Geometry: final body of the model. Coordinates: model frame, mm. Round coordinates to 2 decimals unless told otherwise and drop trailing zeros. Order: outer loops, then holes, each group sorted by start corner. A loop starts at its lowest first (then second) coordinate and runs counter-clockwise, first axis right, second up. Notation, with made-up numbers: M 1.5,11 L 43.5,11 A27 cw 43.5,34 Z; hole C 49.5,25 d1. An arc over 180 degrees is marked long. Return JSON: item names as keys, results as strings. Group by question number.
Q1. Cut plane A-A on z = 285. Output: boundary loops of the cut face in (x, y), and give its area (3 significant figures).
Q2. Ray query, probe 1 along Y at (x, z) = (0, 188.5); probe 2 along Y at (x, z) = (-0.5, 73). Return the intervals inside material, ascending.
Q3. Contact query for flat-ended pins moving along their axis: pin 1 (1.7 mm diameter, centred on x = -3.5, y = 2, fed in from +Z); pin 2 (1.5 mm diameter, centred on x = 0, y = 3.5, fed in from +Z); pin 3 (2.5 mm diameter, centred on y = 0, z = 5.5, fed in from +X); pin 4 (4 mm diameter, centred on y = -2, z = 220.5, fed in from +X). Output: stop coordinate, or through.
```python
from build123d import *
from build123d.topology import SkipClean

# Parameters (mm, degrees)
SKETCH_1_R          = 2.5
EXTRUDE_1_DEPTH     = 345
CUT_EXTRUDE_1_DEPTH = 4.8
SKETCH_3_R          = 5
SKETCH_3_R_2        = 2.75
EXTRUDE_2_DEPTH     = 290
SKETCH_4_R          = 5
EXTRUDE_3_DEPTH     = 5
CUT_EXTRUDE_START   = -5
CUT_EXTRUDE_2_DEPTH = 5


with BuildPart() as part:
    # Sketch 1 → Extrude 1 (new body)
    with BuildSketch(Plane.XY):
        Circle(SKETCH_1_R)
    extrude(amount=EXTRUDE_1_DEPTH)

    # Sketch 2 → Cut-Extrude 1 (cut)
    with BuildSketch(Plane(origin=(0, 0, 3), x_dir=(-1, 0, 0), z_dir=(0, 0, -1))):
        with BuildLine():
            Line((-2, 1.5), (-2, -1.5))
            ThreePointArc((-2, -1.5), (-2.5, 0), (-2, 1.5))
        make_face()
    extrude(amount=-CUT_EXTRUDE_1_DEPTH, mode=Mode.SUBTRACT)



with BuildPart() as body_2:
    # Sketch 3 → Extrude 2 (new body)
    with BuildSketch(Plane.XY.offset(305)):
        Circle(SKETCH_3_R)
        Circle(SKETCH_3_R_2, mode=Mode.SUBTRACT)
    extrude(amount=-EXTRUDE_2_DEPTH)


with BuildPart() as part_1:
    add(part.part)

    add(body_2.part)  # Extrude 3 merges body 2
    # Sketch 4 → Extrude 3 (add)
    with BuildSketch(Plane.XY.offset(305)):
        Circle(SKETCH_4_R)
    extrude(amount=EXTRUDE_3_DEPTH)

    # Sketch 5 → Cut-Extrude 2 (cut)
    with SkipClean():  # the faces are left unmerged after this step: merging them gives an invalid solid
        with BuildSketch(Plane.XY.offset(310).offset(CUT_EXTRUDE_START)):
            with BuildLine():
                Line((-1.5, 4.769696007), (-1.5, 2))
                ThreePointArc((-1.5, 2), (-2.5, 0), (-1.5, -2))
                Line((-1.5, -2), (-1.5, -4.769696007))
                ThreePointArc((-1.5, -4.769696007), (-5, 0), (-1.5, 4.769696007))
            make_face()
            with BuildLine():
                Line((1.5, 4.769696007), (1.5, 2))
                ThreePointArc((1.5, 2), (2.5, 0), (1.5, -2))
                Line((1.5, -2), (1.5, -4.769696007))
                ThreePointArc((1.5, -4.769696007), (5, 0), (1.5, 4.769696007))
            make_face()
        extrude(amount=CUT_EXTRUDE_2_DEPTH, mode=Mode.SUBTRACT)


solid = part_1.part
```
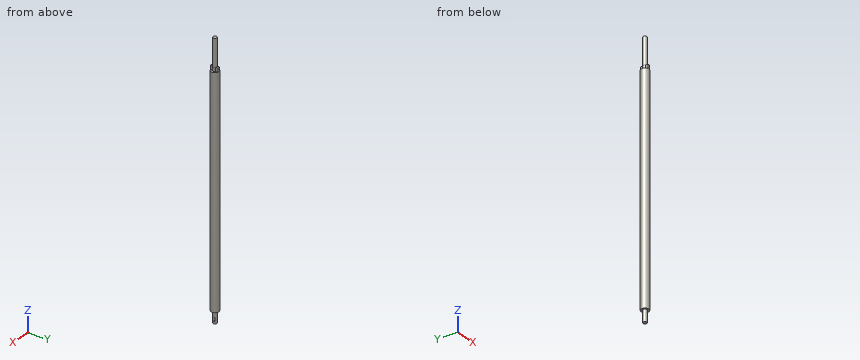
Result sheet:
{
 "1": {"outline": "C 0,0 d10; C 0,0 d5; hole C 0,0 d5.5", "area": "74.4 mm²"},
 "2": {"probe 1": "y = -5 to -2.75, -2.5 to 2.5, 2.75 to 5", "probe 2": "y = -4.97 to -2.7, -2.45 to 2.45, 2.7 to 4.97"},
 "3": {"pin 1": "stops at z = 305", "pin 2": "stops at z = 310", "pin 3": "stops at x = 2", "pin 4": "stops at x = 5"}
}
